```python
from build123d import *

# Parameters (mm, degrees)
SKETCH1_W           = 100
SKETCH1_H           = 50
BOSS_EXTRUDE1_DEPTH = 100
SKETCH2_R           = 51
CUT_EXTRUDE1_DEPTH  = 100
CUT_EXTRUDE2_DEPTH  = 100


with BuildPart() as part:
    # Sketch1 → Boss-Extrude1 (new body)
    with BuildSketch(Plane.XY):
        with Locations((14.926931106, -10.177453027)):
            Rectangle(SKETCH1_W, SKETCH1_H)
    extrude(amount=BOSS_EXTRUDE1_DEPTH)

    # Sketch2 → Cut-Extrude1 (cut)
    with BuildSketch(Plane.ZY.offset(35.073068894)):
        with Locations((144.452221542, -10.177453027)):
            Circle(SKETCH2_R)
    extrude(amount=-CUT_EXTRUDE1_DEPTH, mode=Mode.SUBTRACT)

    # Sketch3 → Cut-Extrude2 (cut)
    with BuildSketch(Plane.XZ.offset(35.177453027)):
        with BuildLine():
            Line((-35.073068894, 80), (-35.073068894, 0))
            Line((-35.073068894, 0), (64.926931106, 0))
            Line((64.926931106, 0), (64.926931106, 80))
            ThreePointArc((64.926931106, 80), (14.926931106, 30), (-35.073068894, 80))
        make_face()
        with BuildLine():
            Line((-27.073068894, 85), (-17.073068894, 85))
            Line((-17.073068894, 85), (-17.073068894, 100))
            Line((-17.073068894, 100), (46.926931106, 100))
            Line((46.926931106, 100), (46.926931106, 85))
            Line((46.926931106, 85), (56.926931106, 85))
            Line((56.926931106, 85), (56.926931106, 80))
            ThreePointArc((56.926931106, 80), (14.926931106, 38), (-27.073068894, 80))
            Line((-27.073068894, 80), (-27.073068894, 85))
        make_face()
    extrude(amount=-CUT_EXTRUDE2_DEPTH, mode=Mode.SUBTRACT)


solid = part.part
```
Work out the finished part from the listing and answer in its coordinate system (mm). A direction names the side the tool comes from. Coordinates: 2 decimals unless noted, no trailing zeros. Order: outer loops, then holes, each group sorted by start corner. A loop starts at its lowest first (then second) coordinate and runs counter-clockwise, first axis right, second up. Notation, with made-up numbers: M 42.5,15 L 86.5,15 A12 cw 86.5,35 Z; hole C -7.75,14 d9. An arc over 180 degrees is marked long. Use CSV: the item, a comma, the result in double quotes.
1) Section A-A on z = 91 is taken. Write down the section's boundary in (x, y).
Worked out:
outline,"M -35.07,-35.18 L -17.07,-35.18 L -17.07,14.82 L -35.07,14.82 Z; M 46.93,-35.18 L 64.93,-35.18 L 64.93,14.82 L 46.93,14.82 Z"
2) For faces 4 (the face through (55.801, -9.812, 93.454)), 5 (the face through (-17.073, -11, 91)), 6 (the face through (56.927, -11, 83)), determine the directions among +Z, -Z, +X, -X, +Y, -Y from which every point of the face is accessible in a straight line to the end or side of a thin tool.
Worked out:
face 4,"+Z, +X, -X"
face 5,"+Z, +Y, -Y"
face 6,"+Y, -Y"
3) Section C-C on z = 63 is taken. Write down the section's boundary in (x, y), plus the area to 3 significant figures.
Worked out:
outline,"M -32.09,-35.18 L -23.48,-35.18 L -23.48,14.82 L -32.09,14.82 Z; M 53.33,-35.18 L 61.95,-35.18 L 61.95,14.82 L 53.33,14.82 Z"
area,"862 mm^2"
4) Determine the mould class of faces 1 (the face through (46.927, -11, 91)), 2 (the face through (64.927, -11, 88)), 3 (the face through (16.026, -10.527, 30.012)) for opening direction X: released by +X, released by -X, zero draft, split by the parting line, or undercut.
Worked out:
face 1,"undercut"
face 2,"released by +X"
face 3,"split by the parting line"
5) Flat-ended cylindrical pins translate along their axes: pin 1 Ø1 at (y, z) = (4.5, 67.5) entering from +X; pin 2 Ø5 at (y, z) = (6, 56.5) entering from -X; pin 3 Ø6 at (x, y) = (3.5, -3) entering from +Z. Find the tip coordinate at first contact, or state that the pin passes through.
Worked out:
pin 1,"stops at x = 63.47"
pin 2,"stops at x = -30.45"
pin 3,"stops at z = 40.56"
6) Section B-B on y = -12.5 is taken. Write down the section's boundary in (x, z).
Worked out:
outline,"M -35.07,80 A50 ccw 64.93,80 L 64.93,93.51 L 46.93,93.51 L 46.93,85 L 56.93,85 L 56.93,80 A42 cw -27.07,80 L -27.07,85 L -17.07,85 L -17.07,93.51 L -35.07,93.51 Z"
7) Section D-D on y = -29 is taken. Write down the section's boundary in (x, z).
Worked out:
outline,"M -35.07,80 A50 ccw 64.93,80 L 64.93,97.05 L 46.93,97.05 L 46.93,85 L 56.93,85 L 56.93,80 A42 cw -27.07,80 L -27.07,85 L -17.07,85 L -17.07,97.05 L -35.07,97.05 Z"
8) Consider line 1 (X direction, y = -1.5, z = 89); line 2 (X direction, y = 0, z = 80); line 3 (Z direction, x = 51, y = -2.5). Determine where each line is inside the solid, lowest interval first. Write a range as [from, to].
Worked out:
line 1,"x = [-35.07, -17.07], [46.93, 64.93]"
line 2,"x = [-35.07, -27.07], [56.93, 64.93]"
line 3,"z = [45.38, 58.49], [85, 94.03]"
